```python
from build123d import *

# Parameters (mm, degrees)
SZKIC2_W                         = 2.5
SZKIC2_H                         = 2.5
SZYK_LINIOWY1_COUNT              = 2
SZYK_LINIOWY1_PITCH              = 5.5
WYTNIJ_WYCI_GNI_CIE1_DEPTH       = 68.915388536
WYTNIJ_WYCI_GNI_CIE1_DEPTH_BACK  = 68.915388536
WYTNIJ_WYCI_GNI_CIE2_DEPTH       = 68.915388602
WYTNIJ_WYCI_GNI_CIE2_DEPTH_BACK  = 68.915388602
SZKIC4_R                         = 6
DODANIE_WYCI_GNI_CIE1_REACH      = 79.915
DODANIE_WYCI_GNI_CIE1_END_RADIUS = 20.5
DODANIE_WYCI_GNI_CIE1_START      = 10
SZKIC5_R                         = 7.5
SZKIC5_R_2                       = 6


# Read off the part's stored shape, not the designer's step: Skorupa1
with BuildPart() as part:
    # Szkic1 → Obrót1 (revolve)
    with BuildSketch(Plane.XY, mode=Mode.PRIVATE) as obr_t1_sk:
        with BuildLine():
            Line((0, 0), (22.5, 0))
            Line((22.5, 0), (22.5, 53.071891388))
            ThreePointArc((22.5, 53.071891388), (11.771243445, 58.228756555), (0, 60))
            Line((0, 60), (0, 0))
        make_face()
    revolve(obr_t1_sk.sketch.rotate(Axis((0, 60, 0), (0, -1, 0)), 180), axis=Axis((0, 60, 0), (0, -1, 0)))

    # Szkic2 → Wycięcie-obrót1 (revolve, cut)
    with BuildSketch(Plane.XY):
        with Locations((21.25, 41.25)):
            Rectangle(SZKIC2_W, SZKIC2_H)
    wyci_cie_obr_t1 = revolve(axis=Axis((0, 43.732823124, 0), (0, 1, 0)), mode=Mode.SUBTRACT)

    # Szyk liniowy1: Wycięcie-obrót1 ×2
    with Locations(*[(0, i * SZYK_LINIOWY1_PITCH, 0) for i in range(1, SZYK_LINIOWY1_COUNT)]):
        add(wyci_cie_obr_t1, mode=Mode.SUBTRACT)

    # Skorupa1 outline → Skorupa1 (revolve, cut)
    with BuildSketch(Plane.XY):
        with BuildLine():
            Line((20.5, 0), (20.5, 38))
            Line((20.5, 38), (18, 38))
            Line((18, 38), (18, 50))
            Line((18, 50), (20.5, 50))
            Line((20.5, 50), (20.500000011, 51.996093505))
            ThreePointArc((20.500000011, 51.996093505), (10.680553516, 56.468147425), (0, 58))
            Line((0, 58), (0, 0))
            Line((0, 0), (20.5, 0))
        make_face()
    revolve(axis=Axis((0, 0, 0), (0, 1, 0)), mode=Mode.SUBTRACT)

    # Szkic3 → Wytnij-wyciągnięcie1 (cut, two sides: drawn at the far end of the back side and taken through both)
    with BuildSketch(Plane.XY.offset(-WYTNIJ_WYCI_GNI_CIE1_DEPTH_BACK)):
        with BuildLine():
            Line((-99.770112831, -131.416252764), (-18, 0))
            ThreePointArc((-18, 0), (0, 10), (18, 0))
            Line((18, 0), (99.770112831, -131.416252764))
            Line((99.770112831, -131.416252764), (99.770112831, -440.974537052))
            Line((99.770112831, -440.974537052), (-99.770112831, -440.974537052))
            Line((-99.770112831, -440.974537052), (-99.770112831, -131.416252764))
        make_face()
    extrude(amount=WYTNIJ_WYCI_GNI_CIE1_DEPTH + WYTNIJ_WYCI_GNI_CIE1_DEPTH_BACK, mode=Mode.SUBTRACT)

    # Szkic4 → Wytnij-wyciągnięcie2 (cut, two sides: drawn at the far end of the back side and taken through both)
    with BuildSketch(Plane.XY.offset(-WYTNIJ_WYCI_GNI_CIE2_DEPTH_BACK)):
        with Locations((0, 30)):
            Circle(SZKIC4_R)
    extrude(amount=WYTNIJ_WYCI_GNI_CIE2_DEPTH + WYTNIJ_WYCI_GNI_CIE2_DEPTH_BACK, mode=Mode.SUBTRACT)

    # Dodanie-wyciągnięcie1: up to this cylinder (the profile starts inside it)
    dodanie_wyci_gni_cie1_end = Plane(origin=(0, 30, 0), z_dir=(0, 1, 0)) * Cylinder(DODANIE_WYCI_GNI_CIE1_END_RADIUS, 201.83, mode=Mode.PRIVATE)
    # Szkic5 → Dodanie-wyciągnięcie1 (add, up to the surface)
    with BuildSketch(Plane.XY.offset(DODANIE_WYCI_GNI_CIE1_START), mode=Mode.PRIVATE) as dodanie_wyci_gni_cie1_sk1:
        with Locations(Location((0, 30, 0), (0, 0, 180))):
            Circle(SZKIC5_R)
        with Locations((0, 30)):
            Circle(SZKIC5_R_2, mode=Mode.SUBTRACT)
    dodanie_wyci_gni_cie1_tool1 = extrude(dodanie_wyci_gni_cie1_sk1.sketch, amount=DODANIE_WYCI_GNI_CIE1_REACH, mode=Mode.PRIVATE) & dodanie_wyci_gni_cie1_end
    dodanie_wyci_gni_cie1 = dodanie_wyci_gni_cie1_tool1.solids().sort_by_distance((7.287868, 30, 10))[0]
    add(dodanie_wyci_gni_cie1)

    # Lustro1: Dodanie-wyciągnięcie1 across plane
    add(dodanie_wyci_gni_cie1.mirror(Plane.XY))


solid = part.part
```
The listing builds one solid part. Answer for the finished solid, in the listing's coordinates (mm). A direction names the side the tool comes from. Coordinates: 2 decimals unless noted, no trailing zeros. Write each loop counter-clockwise with the first axis right and the second up, starting at its lowest first coordinate (ties: lowest second). Pieces come first, ordered by that corner, then holes. Notation, with made-up numbers: (65, 56) - (89, 56) arc R11 cw to (89, 75) - close; hole circle Ø4 at (5.5, -16). An arc over 180 degrees is marked (long way). Return JSON: item names as keys, results as strings. Group by question number.
1. Straight lines are drawn through the part: L1, parallel to Y at x = -6.5, z = 20.5; L2, parallel to X at y = 27.5, z = 0; L3, parallel to Y at x = 0, z = 13. For each, find the intervals that lie inside material, in ascending order.
2. Determine the mould class of faces 1 (the flat face through (-1.4, 50, 18.1)), 2 (the cylindrical face through (17.855, 20.28, 13.691)), 3 (the flat face through (20.1, 42.5, 1.6)) for opening direction Z: released by +Z, released by -Z, zero draft, split by the parting line, or undercut.
3. A cutting plane is placed at B-B, the plane x = 0. Give the number of separate pieces and of enclosed holes in the cut face, plus the area to 3 significant figures.
4. A cutting plane is placed at D-D, the plane y = 15. Determine the outline of the cut face in (x, z).
5. Given pin 1 (4 mm diameter, centred on x = -8.5, y = 27, fed in from -Z); pin 2 (5 mm diameter, centred on x = -7.5, y = 16.5, fed in from -Z); pin 3 (8 mm diameter, centred on x = 8, y = 11, fed in from +Z), each flat-ended and moving along its own axis, determine where each tip first touches the part or whether it passes through.
6. Which of the six approach directions +Z, -Z, +X, -X, +Y, -Y give full straight-line access (tool end or side, diameter ignored) to faces 4 (the flat face through (-2, 24, -10)), 5 (the cylindrical face through (0, 10, -21)), 6 (the flat face through (20.1, 45.5, 1.6))?
7. A cutting plane is placed at A-A, the plane y = 30. Determine the outline of the cut face in (x, z).
Ans:
{
 "1": {"L1": "8.98 to 40, 42.5 to 45.5, 48 to 53.73", "L2": "-22.5 to -20.5, 20.5 to 22.5", "L3": "22.5 to 24, 36 to 37.5, 55.71 to 57.83"},
 "2": {"face 1": "undercut", "face 2": "split by the parting line", "face 3": "zero draft"},
 "3": {"separate pieces": "3", "enclosed holes": "0", "area": "311 mm²"},
 "4": {"outline": "circle Ø45 at (0, 0); hole circle Ø41 at (0, 0)"},
 "5": {"pin 1": "z = -21.54", "pin 2": "z = -21.94", "pin 3": "z = 22.14"},
 "6": {"face 4": "-Y", "face 5": "+Z, -Z, -Y", "face 6": "none"},
 "7": {"outline": "(-7.5, -19.08) arc R20.5 cw to (-7.5, 19.08) - (-7.5, 10) - (-6, 10) - (-6, 21.69) arc R22.5 ccw to (-6, -21.69) - (-6, -10) - (-7.5, -10) - close; (6, -21.69) arc R22.5 ccw to (6, 21.69) - (6, 10) - (7.5, 10) - (7.5, 19.08) arc R20.5 cw to (7.5, -19.08) - (7.5, -10) - (6, -10) - close"}
}
